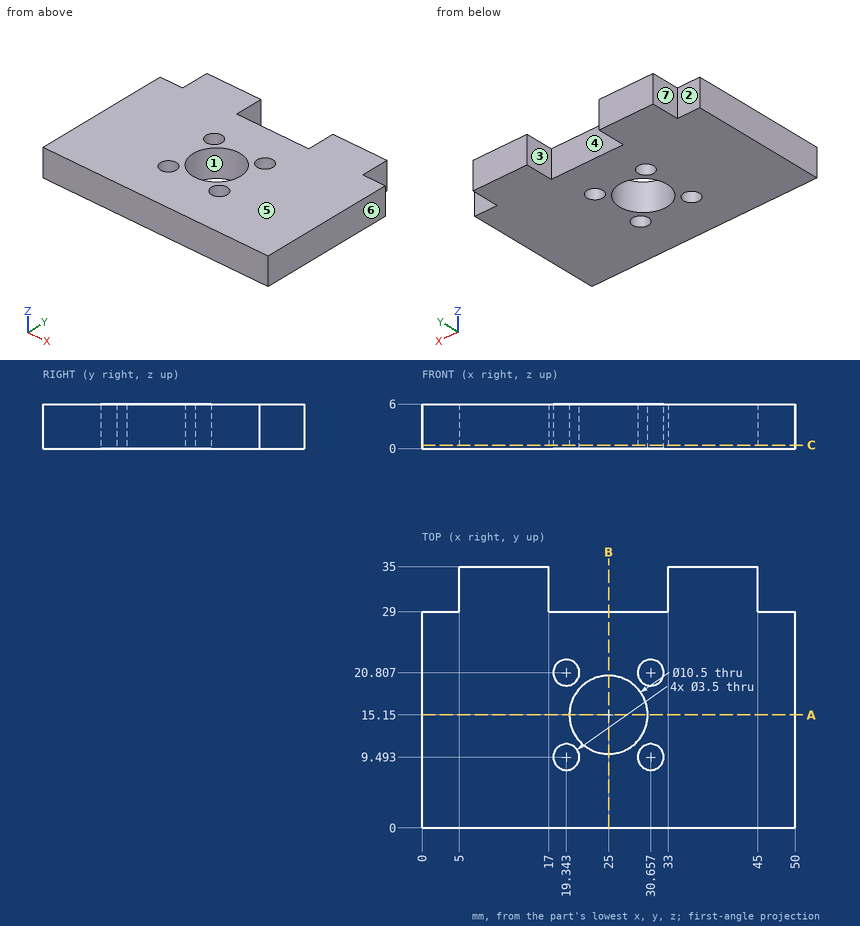
Input: dimensioned drawing with shaded views. Units: mm. Origin: part minimum x, y, z. A direction names the side the tool comes from. Coordinates: 2 decimals unless noted, no trailing zeros. Loops run counter-clockwise (first coordinate to the right, second up) from the corner with the lowest first, then second, coordinate; pieces in that order, holes last. Notation, with made-up numbers: M 21,8 L 79,8 A21 cw 79,16 Z; hole C -16,61.5 d2. An arc over 180 degrees is marked long. Use a Markdown table: item, result. Add a question column.
1) Section B-B, the plane x = 25. Return the cut outline in (y, z), plus the area to 3 significant figures.
2) Section A-A, the plane y = 15.15. Return the cut outline in (x, z).
3) Section C-C, the plane z = 0.5. Return the cut outline in (x, y).
4) Pin query (flat end, axial travel): P1, Ø2.5, axis at x = 48.5, z = 3.5, coming from the +Y side; P2, Ø1.8, axis at y = 33.5, z = 4, coming from the +X side; P3, Ø1.8, axis at y = 32.5, z = 4.5, coming from the -X side; P4, Ø6.5, axis at x = 25, y = 15.15, coming from the -Z side. Return the tip coordinate at first contact, or that it passes through.
5) Set-up query: the marked faces 1, 2 and 3. Return all of +Z, -Z, +X, -X, +Y, -Y with unobstructed straight access to the full face (end or side cutting, diameter ignored); none if empty.
6) Line query: L1, parallel to X at y = 32, z = 2.95; L2, parallel to Y at x = 21.5, z = 5.75; L3, parallel to Y at x = 25, z = 4. Output: solid intervals per line, ascending. Write a range as from..to.
7) Draft query along X for the marked faces 4, 5, 6 and 7. Return one class per face: +X half, -X half, draft (parallel to the pull), parting line (faces both ways), or undercut.
Answer below:
| question | item | result |
|---|---|---|
| 1 | outline | M 0,0 L 9.9,0 L 9.9,6 L 0,6 Z; M 20.4,0 L 29,0 L 29,6 L 20.4,6 Z |
| 1 | area | 111 mm2 |
| 2 | outline | M 0,0 L 19.75,0 L 19.75,6 L 0,6 Z; M 30.25,0 L 50,0 L 50,6 L 30.25,6 Z |
| 3 | outline | M 0,0 L 50,0 L 50,29 L 45,29 L 45,35 L 33,35 L 33,29 L 17,29 L 17,35 L 5,35 L 5,29 L 0,29 Z; hole C 19.34,9.49 d3.5; hole C 19.34,20.81 d3.5; hole C 25,15.15 d10.5; hole C 30.66,9.49 d3.5; hole C 30.66,20.81 d3.5 |
| 4 | P1 | y = 29 |
| 4 | P2 | x = 45 |
| 4 | P3 | x = 5 |
| 4 | P4 | through |
| 5 | face 1 | +Z, -Z |
| 5 | face 2 | +Z, -Z, -X, +Y |
| 5 | face 3 | +Z, -Z, +Y |
| 6 | L1 | 5..17, 33..45 |
| 6 | L2 | 0..11.24, 19.06..29 |
| 6 | L3 | 0..9.9, 20.4..29 |
| 7 | face 4 | undercut |
| 7 | face 5 | draft |
| 7 | face 6 | +X half |
| 7 | face 7 | -X half |
